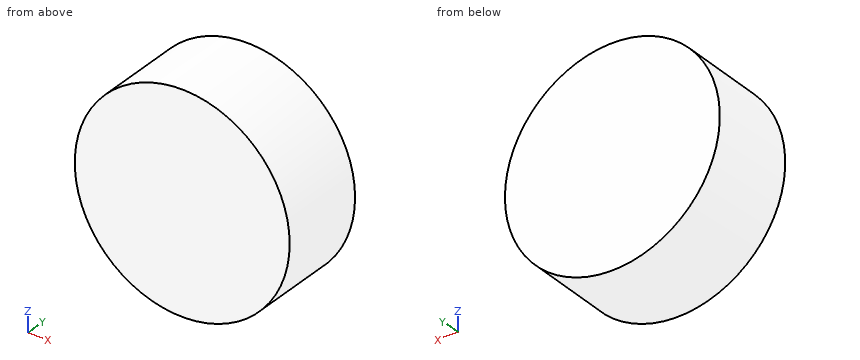
```python
from build123d import *

# Parameters (mm, degrees)
F0_R     = 19.05
F1_DEPTH = 15.875
F2_R     = 9.525
F3_DEPTH = 12.7
F4_DEPTH = 12.7


with BuildPart() as f1:
    # F0 (on Front) → F1 (new body)
    with BuildSketch(Plane.XZ):
        Circle(F0_R)
    extrude(amount=F1_DEPTH)

    # F2 (on Front) → F3 (cut)
    with BuildSketch(Plane.XZ):
        Circle(F2_R)
    extrude(amount=-F3_DEPTH, mode=Mode.SUBTRACT)

    # F2 (on Front) → F4 (cut)
    with BuildSketch(Plane.XZ):
        Circle(F2_R)
    extrude(amount=-F4_DEPTH, mode=Mode.SUBTRACT)


solid = f1.part
```
Build history of the part. All positions in model axes, mm. Give positions to 0.01 mm unless a question says otherwise; leave off trailing zeros. Loops run counter-clockwise (first coordinate to the right, second up) from the corner with the lowest first, then second, coordinate; pieces in that order, holes last. Notation, with made-up numbers: (51.25, -15) - (68.25, -15) arc R25 ccw to (68.25, 11) - close; hole circle Ø5 at (71.25, 68). An arc over 180 degrees is marked (long way). Use a Markdown table: item, result.
(1) Wall check: line 1 along X through (y, z) = (-13, -0.5); line 2 along Z through (x, y) = (11, -9.75). Give the ranges that are in metal, low to high.
Taken from the geometry:
| item | result |
|---|---|
| line 1 | -19.04 to 19.04 |
| line 2 | -15.55 to 15.55 |
(2) Band-saw the part on C-C (z = -15). Give the cut face in (x, y) (3 decimals), and give its area (3 significant figures).
Taken from the geometry:
| item | result |
|---|---|
| outline | (-11.743, -15.875) - (11.743, -15.875) - (11.743, 0) - (-11.743, 0) - close |
| area | 373 mm2 |
(3) Band-saw the part on B-B (x = -8). Give the cut face in (y, z) (3 decimals), and give its area (3 significant figures).
Taken from the geometry:
| item | result |
|---|---|
| outline | (-15.875, -17.289) - (0, -17.289) - (0, 17.289) - (-15.875, 17.289) - close |
| area | 549 mm2 |
(4) Band-saw the part on A-A (y = -7.5). Give the cut face in (x, z).
Taken from the geometry:
| item | result |
|---|---|
| outline | circle Ø38.1 at (0, 0) |
(5) Drop flat-ended pins along their axis: pin 1 Ø8 at (x, y) = (-13, -7.5) entering from +Z; pin 2 Ø4 at (x, y) = (-9, -6.5) entering from -Z; pin 3 Ø2 at (y, z) = (-2, 2) entering from +X. Give the stop position or say it passes through.
Taken from the geometry:
| item | result |
|---|---|
| pin 1 | z = 16.79 |
| pin 2 | z = -17.72 |
| pin 3 | x = 19.02 |
